Geometry check sheet. Reference: the model listing, model coordinates, mm. A direction names the side the tool comes from. Round coordinates to 2 decimals unless told otherwise and drop trailing zeros. Write each loop counter-clockwise with the first axis right and the second up, starting at its lowest first coordinate (ties: lowest second). Pieces come first, ordered by that corner, then holes. Notation, with made-up numbers: (59, 19) -> (98, 19) arc R30 ccw to (98, 53) -> close; hole circle Ø4 at (-22, -5). An arc over 180 degrees is marked (long way). Put each result on its own line as item: value. Start each with the question number.
from build123d import *

# Parameters (mm, degrees)
SKETCH1_R           = 1.5
BOSS_EXTRUDE1_DEPTH = 17
SKETCH2_W           = 20
SKETCH2_H           = 4
CUT_EXTRUDE1_DEPTH  = 4


with BuildPart() as part:
    # Sketch1 → Boss-Extrude1 (new body)
    with BuildSketch(Plane(origin=(0, 0, 0), x_dir=(1, 0, 0), z_dir=(0, 1, 0))):
        with BuildLine():
            Line((-3, 0), (-67, 0))
            ThreePointArc((-67, 0), (-69.121320344, 0.878679656), (-70, 3))
            Line((-70, 3), (-70, 50))
            ThreePointArc((-70, 50), (-69.121320344, 52.121320344), (-67, 53))
            Line((-67, 53), (-3, 53))
            ThreePointArc((-3, 53), (-0.878679656, 52.121320344), (0, 50))
            Line((0, 50), (0, 3))
            ThreePointArc((0, 3), (-0.878679656, 0.878679656), (-3, 0))
        make_face()
        with Locations(Location((-67, 50, 0), (0, 0, 270))):
            Circle(SKETCH1_R, mode=Mode.SUBTRACT)
        with Locations(Location((-3, 50, 0), (0, 0, 90))):
            Circle(SKETCH1_R, mode=Mode.SUBTRACT)
        with Locations(Location((-3, 3, 0), (0, 0, 270))):
            Circle(SKETCH1_R, mode=Mode.SUBTRACT)
        with Locations(Location((-67, 3, 0), (0, 0, 90))):
            Circle(SKETCH1_R, mode=Mode.SUBTRACT)
        Polygon((-66, 46.5), (-63.5, 49), (-6.5, 49), (-4, 46.5), (-4, 6.5), (-6.5, 4), (-63.5, 4), (-66, 6.5), align=None, mode=Mode.SUBTRACT)
    extrude(amount=BOSS_EXTRUDE1_DEPTH)

    # Sketch2 → Cut-Extrude1 (cut)
    with BuildSketch(Plane.ZY.offset(70)):
        with Locations((-26.5, 2)):
            Rectangle(SKETCH2_W, SKETCH2_H)
    extrude(amount=-CUT_EXTRUDE1_DEPTH, mode=Mode.SUBTRACT)


solid = part.part
(1) Sectioned sample at D-D (y = 2.5). Record the cut outline in (x, z).
(2) Mould release check, pull along X, two halves, no side actions. Record for faces 4 (the flat face through (-35, 8, -53)), 5 (the flat face through (0, 8, -27)), 6 (the flat face through (-35, 8, -4)): +X half, -X half, draft (parallel to the pull), parting line (faces both ways), or undercut.
(3) Sectioned sample at A-A (x = -9). Record the cut outline in (y, z).
(4) Sectioned sample at C-C (y = 6.25). Record the cut outline in (x, z), and give its area (4 significant figures).
(5) Go/stop test with flat-tipped pins: pin 1 Ø3 at (x, z) = (-68.5, -22.5) entering from -Y; pin 2 Ø2.5 at (x, z) = (-67, -50) entering from -Y. Record where each tip stops, or that it passes through.
(6) Material ranges on L1, parallel to X at y = 11.5, z = -50; L2, parallel to Z at x = -28.5, y = 9.25; L3, parallel to X at y = 6, z = -39, recorded low to high. Write a range as from..to.
(7) Set-up check for faces 1 (the flat face through (-66, 8, -26)), 2 (the cylindrical face through (-0.86, 8.38, -0.9)), 3 (the flat face through (-68, 4, -27)): record each of +Z, -Z, +X, -X, +Y, -Y from which the full face is reachable in a straight line by a thin tool's end or side.
(8) Sectioned sample at B-B (z = -22). Record the cut outline in (x, y).
Found:
1. outline: (-70, -50) arc R3 ccw to (-67, -53) -> (-3, -53) arc R3 ccw to (0, -50) -> (0, -3) arc R3 ccw to (-3, 0) -> (-67, 0) arc R3 ccw to (-70, -3) -> (-70, -16.5) -> (-66, -16.5) -> (-66, -6.5) -> (-63.5, -4) -> (-6.5, -4) -> (-4, -6.5) -> (-4, -46.5) -> (-6.5, -49) -> (-63.5, -49) -> (-66, -46.5) -> (-66, -36.5) -> (-70, -36.5) -> close; hole circle Ø3 at (-67, -50); hole circle Ø3 at (-67, -3); hole circle Ø3 at (-3, -50); hole circle Ø3 at (-3, -3)
2. face 4: draft
2. face 5: +X half
2. face 6: undercut
3. outline: (0, -53) -> (17, -53) -> (17, -49) -> (0, -49) -> close; (0, -4) -> (17, -4) -> (17, 0) -> (0, 0) -> close
4. outline: (-70, -50) arc R3 ccw to (-67, -53) -> (-3, -53) arc R3 ccw to (0, -50) -> (0, -3) arc R3 ccw to (-3, 0) -> (-67, 0) arc R3 ccw to (-70, -3) -> close; hole circle Ø3 at (-67, -50); hole circle Ø3 at (-67, -3); hole (-66, -46.5) -> (-63.5, -49) -> (-6.5, -49) -> (-4, -46.5) -> (-4, -6.5) -> (-6.5, -4) -> (-63.5, -4) -> (-66, -6.5) -> close; hole circle Ø3 at (-3, -50); hole circle Ø3 at (-3, -3)
4. area: 896.5 mm2
5. pin 1: y = 4
5. pin 2: through
6. L1: -70..-68.5, -65.5..-4.5, -1.5..0
6. L2: -53..-49, -4..0
6. L3: -70..-66, -4..0
7. face 1: +Y, -Y
7. face 2: +Z, +X, +Y, -Y
7. face 3: -X, -Y
8. outline: (-70, 4) -> (-66, 4) -> (-66, 17) -> (-70, 17) -> close; (-4, 0) -> (0, 0) -> (0, 17) -> (-4, 17) -> close
